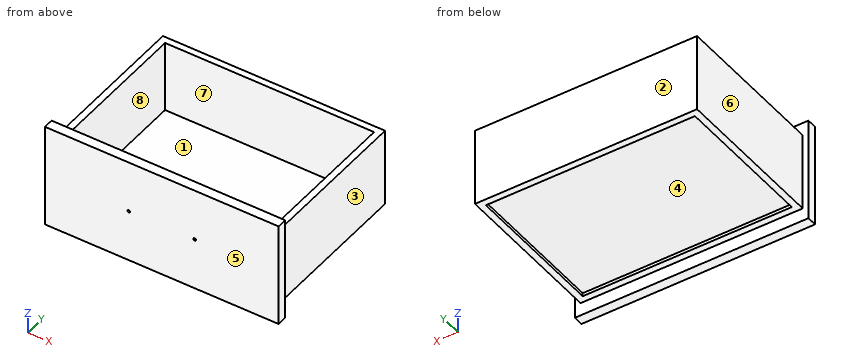
```python
from build123d import *

# Parameters (mm, degrees)
F0_W     = 431.8
F0_H     = 304.8
F0_W_2   = 406.4
F0_H_2   = 279.4
F1_DEPTH = 152.4
F2_W     = 279.4
F2_H     = 6.35
F3_DEPTH = 406.4
F4_W     = 454.152
F4_H     = 203.2
F5_DEPTH = 19.05
F7_D     = 5.0038
F7_DEPTH = 31.75


with BuildPart() as f1:
    # F0 (on Top) → F1 (new body)
    with BuildSketch(Plane.XY):
        Rectangle(F0_W, F0_H)
        Rectangle(F0_W_2, F0_H_2, mode=Mode.SUBTRACT)
    extrude(amount=F1_DEPTH)

    # F2 (on face) → F3 (join, through all)
    with BuildSketch(Plane.YZ.offset(-203.2)):
        with Locations((0, 9.525)):
            Rectangle(F2_W, F2_H)
    extrude(amount=F3_DEPTH)

    # F4 (on face) → F5 (join)
    with BuildSketch(Plane.XZ.offset(152.4)):
        with Locations((0, 76.2)):
            Rectangle(F4_W, F4_H)
    extrude(amount=F5_DEPTH)

    # F7
    with Locations(Plane.XZ.offset(171.45)):
        with Locations((-64.008, 76.2), (64.008, 76.2)):
            Hole(F7_D / 2, depth=F7_DEPTH)


solid = f1.part
```
Geometry check sheet. Reference: the model listing, model coordinates, mm. Face numbers are marked on the shaded views. A direction names the side the tool comes from. Coordinates: 2 decimals unless noted, no trailing zeros. Order: outer loops, then holes, each group sorted by start corner. A loop starts at its lowest first (then second) coordinate and runs counter-clockwise, first axis right, second up. Notation, with made-up numbers: (-25.5, -30) - (28.5, -30) arc R21 cw to (28.5, -9) - close; hole circle Ø10 at (-21, 17.5). An arc over 180 degrees is marked (long way). Answer as a JSON object with one key per item and string values. Group by question number.
Item 1: Draft check along Y on the marked faces 5, 6, 7 and 8. Enter one of: +Y half, -Y half, draft (parallel to the pull), parting line (faces both ways), or undercut.
Item 2: Scan lines: probe 1 along X at (y, z) = (-164, 76); probe 2 along X at (y, z) = (17, 1); probe 3 along Y at (x, z) = (107, 39). Record each from-to range of solid material in increasing order.
Item 3: Sectioned sample at C-C, the plane y = 108.5. Record the cut outline in (x, z), and give its area (3 significant figures).
Item 4: Sectioned sample at A-A, the plane z = 142. Record the cut outline in (x, y).
Item 5: Tool access check on the marked faces 1, 2, 3 and 4. Record the directions out of +Z, -Z, +X, -X, +Y, -Y that give a thin tool (end or side, any length) a straight path to the whole face; none if there is none.
Item 6: Sectioned sample at B-B, the plane x = 15.5. Record the cut outline in (y, z), and give its area (3 significant figures).
Item 7: Depth check by flat-ended pin: pin 1 Ø7 at (y, z) = (-47.5, 3) entering from -X; pin 2 Ø8 at (x, y) = (3, 35) entering from -Z; pin 3 Ø5 at (y, z) = (-51, 3) entering from +X. Enter the tip coordinate at first touch or a pass-through.
Resolved:
{
 "1": {"face 5": "-Y half", "face 6": "draft", "face 7": "undercut", "face 8": "undercut"},
 "2": {"probe 1": "-227.08 to -66.5, -61.51 to 61.51, 66.5 to 227.08", "probe 2": "-215.9 to -203.2, 203.2 to 215.9", "probe 3": "-171.45 to -139.7, 139.7 to 152.4"},
 "3": {"outline": "(-215.9, 0) - (-203.2, 0) - (-203.2, 6.35) - (203.2, 6.35) - (203.2, 0) - (215.9, 0) - (215.9, 152.4) - (203.2, 152.4) - (203.2, 12.7) - (-203.2, 12.7) - (-203.2, 152.4) - (-215.9, 152.4) - close", "area": "6,450 mm^2"},
 "4": {"outline": "(-227.08, -171.45) - (227.08, -171.45) - (227.08, -152.4) - (215.9, -152.4) - (215.9, 152.4) - (-215.9, 152.4) - (-215.9, -152.4) - (-227.08, -152.4) - close; hole (-203.2, -139.7) - (203.2, -139.7) - (203.2, 139.7) - (-203.2, 139.7) - close"},
 "5": {"face 1": "+Z", "face 2": "+Z, -Z, +X, -X, +Y", "face 3": "+Z, -Z, +X, +Y", "face 4": "-Z"},
 "6": {"outline": "(-171.45, -25.4) - (-152.4, -25.4) - (-152.4, 0) - (-139.7, 0) - (-139.7, 6.35) - (139.7, 6.35) - (139.7, 0) - (152.4, 0) - (152.4, 152.4) - (139.7, 152.4) - (139.7, 12.7) - (-139.7, 12.7) - (-139.7, 152.4) - (-152.4, 152.4) - (-152.4, 177.8) - (-171.45, 177.8) - close", "area": "9,520 mm^2"},
 "7": {"pin 1": "x = -215.9", "pin 2": "z = 6.35", "pin 3": "x = 215.9"}
}
